Print and shaded views of the part. All mm, measured from the part's lowest x, y and z. A direction names the side the tool comes from. Round coordinates to 2 decimals unless told otherwise and drop trailing zeros. Order: outer loops, then holes, each group sorted by start corner. A loop starts at its lowest first (then second) coordinate and runs counter-clockwise, first axis right, second up. Notation, with made-up numbers: (37.25, 53) - (85.25, 53) arc R31 cw to (85.25, 87) - close; hole circle Ø4 at (16, 85). An arc over 180 degrees is marked (long way). Write item = value, one per line.
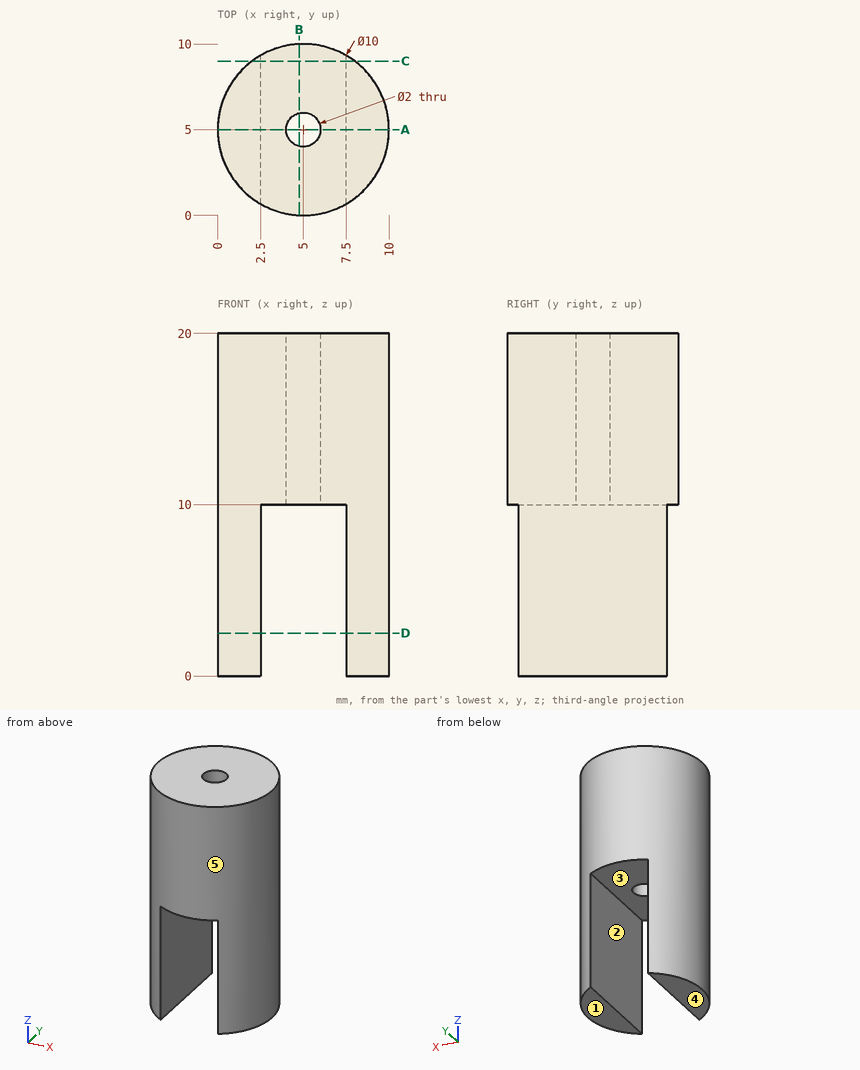
(1) Drop flat-ended pins along their axis: pin 1 (2.5 mm diameter, centred on x = 6, y = 6.5, fed in from -Z); pin 2 (3 mm diameter, centred on x = 8.5, z = 6, fed in from +Y); pin 3 (3 mm diameter, centred on y = 7.5, z = 14.5, fed in from +X). Give the stop position or say it passes through.
Solved:
pin_1 = 10
pin_2 = 9.33
pin_3 = 9.9
(2) Band-saw the part on D-D on z = 2.5. List the corners of the cut face in (x, y).
Solved:
outline = (2.5, 0.67) - (2.5, 9.33) arc R5 ccw to start; (7.5, 0.67) arc R5 ccw to (7.5, 9.33) - close
(3) Band-saw the part on C-C on y = 9. List the corners of the cut face in (x, z).
Solved:
outline = (2, 0) - (2.5, 0) - (2.5, 10) - (7.5, 10) - (7.5, 0) - (8, 0) - (8, 20) - (2, 20) - close
(4) Band-saw the part on A-A on y = 5. List the corners of the cut face in (x, z), plus the area to 3 significant figures.
Solved:
outline = (0, 0) - (2.5, 0) - (2.5, 10) - (4, 10) - (4, 20) - (0, 20) - close; (6, 10) - (7.5, 10) - (7.5, 0) - (10, 0) - (10, 20) - (6, 20) - close
area = 130 mm²
(5) Probe line 1 along X through (y, z) = (2.5, 4.5); line 2 along Y through (x, z) = (5, 15.5); line 3 along Z through (x, y) = (6, 7). List the from-to ranges inside material, lowest first.
Solved:
line_1 = 0.67 to 2.5, 7.5 to 9.33
line_2 = 0 to 4, 6 to 10
line_3 = 10 to 20
(6) Tool access for the marked faces 1 and 2: list every direction of +Z, -Z, +X, -X, +Y, -Y with a clear straight run to the whole face (end or side of a thin tool).
Solved:
face_1 = -Z, +X, -X, +Y, -Y
face_2 = -Z, +Y, -Y
(7) Band-saw the part on B-B on x = 4.75. List the corners of the cut face in (y, z), plus the area to 3 significant figures.
Solved:
outline = (0.01, 10) - (4.03, 10) - (4.03, 20) - (0.01, 20) - close; (5.97, 10) - (9.99, 10) - (9.99, 20) - (5.97, 20) - close
area = 80.5 mm²
(8) Pull direction X, two halves, no side cores. Call the marked faces 3, 4 and 5: released by +X, released by -X, zero draft, split by the parting line, or undercut.
Solved:
face_3 = undercut
face_4 = zero draft
face_5 = split by the parting line
